The figure shows three views and two pictorial views of one solid part (mm, origin at its lowest corner). Answer the questions. A direction names the side the tool comes from. Coordinates: 2 decimals unless noted, no trailing zeros. Order: outer loops, then holes, each group sorted by start corner. A loop starts at its lowest first (then second) coordinate and runs counter-clockwise, first axis right, second up. Notation, with made-up numbers: (6, -31.5) - (33, -31.5) arc R29 ccw to (33, 2.5) - close; hole circle Ø11 at (1, 10). An arc over 180 degrees is marked (long way). Use one line per item in the form item = value.
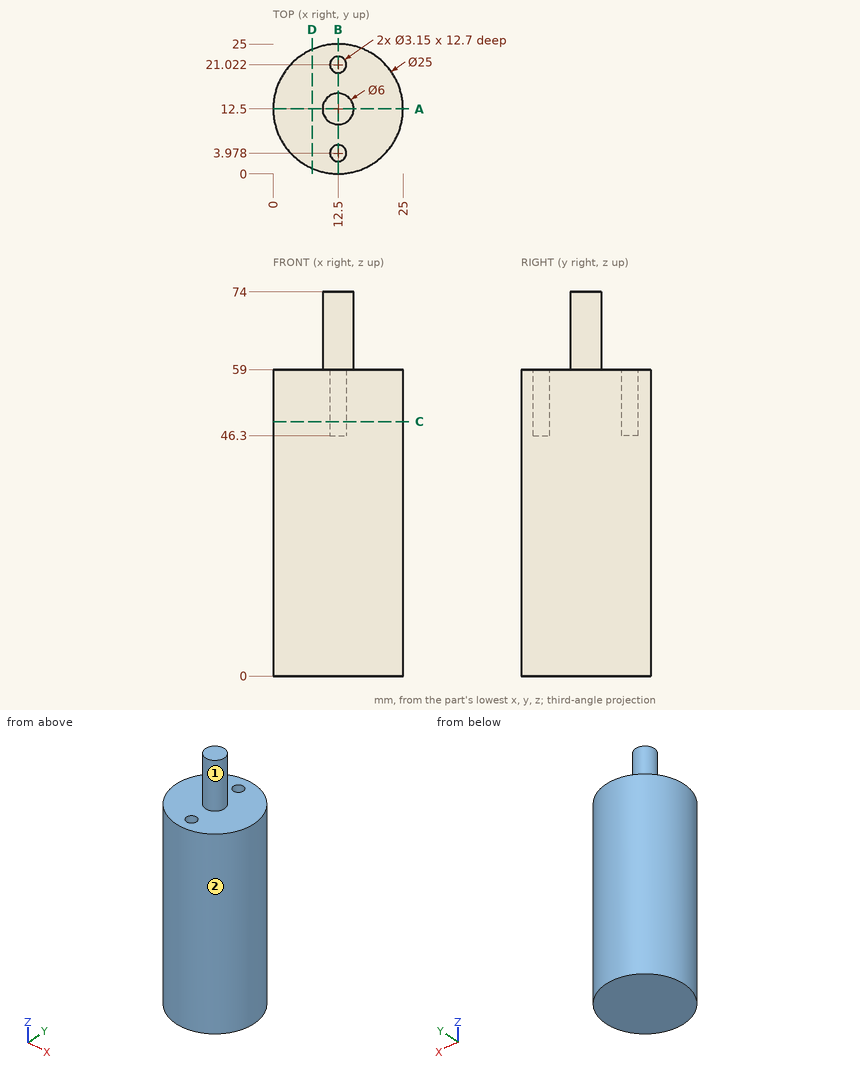
(1) Straight lines are drawn through the part: L1, parallel to Y at x = 12.5, z = 56; L2, parallel to Z at x = 19.75, y = 10.25; L3, parallel to Y at x = 13.25, z = 56.5. For each, find the intervals that lie inside material, in ascending order.
Answer list:
L1 = 0 to 2.4, 5.55 to 19.45, 22.6 to 25
L2 = 0 to 59
L3 = 0.02 to 2.59, 5.36 to 19.64, 22.41 to 24.98
(2) Section A-A, the plane y = 12.5 is taken. Write down the section's boundary in (x, z), then the cut area to 4 significant figures.
Answer list:
outline = (0, 0) - (25, 0) - (25, 59) - (15.5, 59) - (15.5, 74) - (9.5, 74) - (9.5, 59) - (0, 59) - close
area = 1,565 mm2
(3) Section B-B, the plane x = 12.5 is taken. Write down the section's boundary in (y, z), then the cut area to 4 significant figures.
Answer list:
outline = (0, 0) - (25, 0) - (25, 59) - (22.6, 59) - (22.6, 46.3) - (19.45, 46.3) - (19.45, 59) - (15.5, 59) - (15.5, 74) - (9.5, 74) - (9.5, 59) - (5.55, 59) - (5.55, 46.3) - (2.4, 46.3) - (2.4, 59) - (0, 59) - close
area = 1,485 mm2
(4) Section C-C, the plane z = 49 is taken. State how many separate pieces and enclosed holes the cut face has, then the cut area to 3 significant figures.
Answer list:
separate_pieces = 1
enclosed_holes = 2
area = 475 mm2
(5) Which of the six approach directions +Z, -Z, +X, -X, +Y, -Y give full straight-line access (tool end or side, diameter ignored) to the marked faces 1 and 2?
Answer list:
face_1 = +Z
face_2 = +Z, -Z
(6) Given pin 1 Ø3.5 at (x, y) = (12, 22) entering from +Z; pin 2 Ø0.9 at (x, y) = (12.5, 4.5) entering from +Z; pin 3 Ø1 at (y, z) = (14.5, 14) entering from -X, each flat-ended and moving along its own axis, determine where each tip first touches the part or whether it passes through.
Answer list:
pin_1 = 59
pin_2 = 46.3
pin_3 = 0.09
(7) Section D-D, the plane x = 7.5 is taken. Write down the section's boundary in (y, z).
Answer list:
outline = (1.04, 0) - (23.96, 0) - (23.96, 59) - (1.04, 59) - close
